CAD build for the part. Positions are in the model's coordinates, mm. Face numbers are marked on the shaded views. A direction names the side the tool comes from. Round coordinates to 2 decimals unless told otherwise and drop trailing zeros. Loops run counter-clockwise (first coordinate to the right, second up) from the corner with the lowest first, then second, coordinate; pieces in that order, holes last. Notation, with made-up numbers: (-28, -19) - (-19, -19) arc R15 ccw to (-19, -7) - close; hole circle Ø6 at (39, 0). An arc over 180 degrees is marked (long way). Use one line per item in the form item = value.
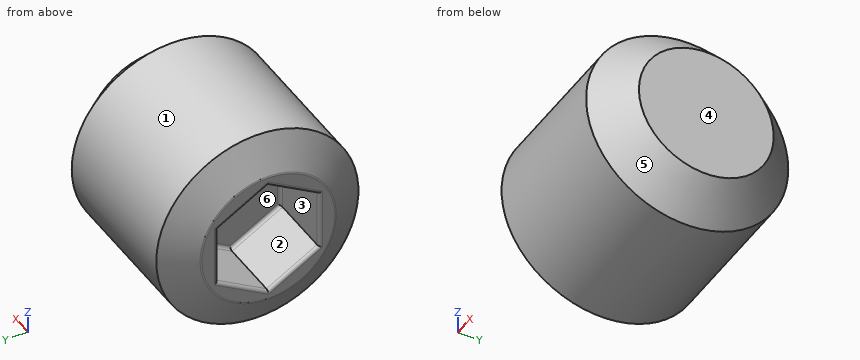
from build123d import *

# Parameters (mm, degrees)
CUT_EXTRUDE_1_DEPTH = 2
CHAMFER_1_SIZE      = 1
CHAMFER_1_SIZE2     = 0.577350269
FILLET_1_R          = 0.1


with BuildPart() as part:
    # Эскиз1 → Повернуть1 (revolve)
    with BuildSketch(Plane(origin=(0, 0, 0), x_dir=(-1, 0, 0), z_dir=(0, 0, -1))):
        Polygon((-6, 2), (-6, 0), (0, 0), (0, 3), (-5, 3), align=None)
    revolve(axis=Axis((6, 0, 0), (-1, 0, 0)))

    # Эскиз2 → Вырез-Вытянуть1 (cut)
    with BuildSketch(Plane.ZY):
        Polygon((1.732050808, 0), (0.866025404, 1.5), (-0.866025404, 1.5), (-1.732050808, 0), (-0.866025404, -1.5), (0.866025404, -1.5), align=None)
    extrude(amount=-CUT_EXTRUDE_1_DEPTH, mode=Mode.SUBTRACT)

    # Фаска1
    chamfer_1_edges = [part.edges().sort_by_distance(p)[0] for p in [
        (0, -3, 0),
    ]]
    chamfer_1_side = [part.faces().sort_by_distance(p)[0] for p in [
        (0, -2.915147186, 0),
    ]]
    chamfer(chamfer_1_edges, length=CHAMFER_1_SIZE, length2=CHAMFER_1_SIZE2, reference=chamfer_1_side[0])

    # Скругление1
    fillet_1_edges = [part.edges().sort_by_distance(p)[0] for p in [
        (2, -0.75, 1.299038106),
        (2, -1.5, 0),
        (2, -0.75, -1.299038106),
        (2, 0.75, -1.299038106),
        (2, 1.5, 0),
        (2, 0.75, 1.299038106),
        (0, -0.75, 1.299038106),
        (0, 0.75, 1.299038106),
        (0, 1.5, 0),
        (0, 0.75, -1.299038106),
        (0, -0.75, -1.299038106),
        (0, -1.5, 0),
        (0, -2, 0),
    ]]
    fillet(fillet_1_edges, radius=FILLET_1_R)


solid = part.part
1) Drill centre lines: probe 1 along Z at (x, y) = (1.45, -1.4); probe 2 along Z at (x, y) = (1.1, -0.25); probe 3 along X at (y, z) = (0.7, -0.8). Where is each one in solid material? Low to high.
Report:
probe_1 = -2.65 to -0.92, 0.92 to 2.65
probe_2 = -2.99 to -1.59, 1.59 to 2.99
probe_3 = 2 to 6
2) Flat gauge pins, fed straight in: pin 1 (1.9 mm diameter, centred on x = 0.5, z = 0.5, fed in from -Y); pin 2 (1.4 mm diameter, centred on y = -0.5, z = 0.5, fed in from -X); pin 3 (3 mm diameter, centred on x = 4.5, y = 2, fed in from +Z). Where does each tip first touch, or does it go through?
Report:
pin_1 = -3
pin_2 = 2
pin_3 = 2.96
3) Slice it at C-C (x = 3.95). Write the cut outline in (y, z).
Report:
outline = circle Ø6 at (0, 0)
4) Two-plate mould, pull along Z, no slides. Class the marked faces 1, 2, 3 and 4: +Z half, -Z half, draft (parallel to the pull), parting line (faces both ways), or undercut.
Report:
face_1 = parting line
face_2 = undercut
face_3 = undercut
face_4 = draft
5) Tool access for the marked faces 5 and 6: list every direction of +Z, -Z, +X, -X, +Y, -Y with a clear straight run to the whole face (end or side of a thin tool).
Report:
face_5 = +X
face_6 = -X
6) Slice it at B-B (z = 0). Write the cut outline in (x, y).
Report:
outline = (0, -1.97) arc R0.1 ccw to (0.01, -2.02) - (0.58, -3) - (5, -3) - (6, -2) - (6, 2) - (5, 3) - (0.58, 3) - (0.01, 2.02) arc R0.1 ccw to (0, 1.97) - (0, 1.6) arc R0.1 ccw to (0.1, 1.5) - (1.9, 1.5) arc R0.1 cw to (2, 1.4) - (2, -1.4) arc R0.1 cw to (1.9, -1.5) - (0.1, -1.5) arc R0.1 ccw to (0, -1.6) - close
7) Slice it at A-A (x = 1.7). Write the cut outline in (y, z).
Report:
outline = circle Ø6 at (0, 0); hole (-1.5, -0.87) - (0, -1.73) - (1.5, -0.87) - (1.5, 0.87) - (0, 1.73) - (-1.5, 0.87) - close
